Can you work these out from the model? Positions are in its coordinate system, mm. A direction names the side the tool comes from. Give positions to 0.01 mm unless a question says otherwise; leave off trailing zeros. Write each loop counter-clockwise with the first axis right and the second up, starting at its lowest first coordinate (ties: lowest second). Pieces come first, ordered by that corner, then holes.
from build123d import *

# Parameters (mm, degrees)
SKETCH1_R           = 2.3
BOSS_EXTRUDE1_DEPTH = 10


with BuildPart() as part:
    # Sketch1 → Boss-Extrude1 (new body)
    with BuildSketch(Plane.XY):
        with BuildLine():
            Line((14.271948898, -9.838051102), (14.061948898, -9.628051102))
            Line((14.061948898, -9.628051102), (14.271948898, -9.418051102))
            Line((14.271948898, -9.418051102), (14.271948898, -6.788711274))
            Line((14.271948898, -6.788711274), (16.932609069, -4.128051102))
            Line((16.932609069, -4.128051102), (18.571948898, -4.128051102))
            Line((18.571948898, -4.128051102), (18.571948898, -6.233051102))
            Line((18.571948898, -6.233051102), (19.186948898, -6.233051102))
            Line((19.186948898, -6.233051102), (20.371948898, -5.048051102))
            Line((20.371948898, -5.048051102), (20.371948898, 5.791948898))
            Line((20.371948898, 5.791948898), (19.186948898, 6.976948898))
            Line((19.186948898, 6.976948898), (18.571948898, 6.976948898))
            Line((18.571948898, 6.976948898), (18.571948898, 4.871948898))
            Line((18.571948898, 4.871948898), (16.932609069, 4.871948898))
            Line((16.932609069, 4.871948898), (14.271948898, 7.532609069))
            Line((14.271948898, 7.532609069), (14.271948898, 10.161948898))
            Line((14.271948898, 10.161948898), (14.061948898, 10.371948898))
            Line((14.061948898, 10.371948898), (14.271948898, 10.581948898))
            Line((14.271948898, 10.581948898), (14.271948898, 13.211288726))
            Line((14.271948898, 13.211288726), (16.932609069, 15.871948898))
            Line((16.932609069, 15.871948898), (18.571948898, 15.871948898))
            Line((18.571948898, 15.871948898), (18.571948898, 13.766948898))
            Line((18.571948898, 13.766948898), (19.186948898, 13.766948898))
            Line((19.186948898, 13.766948898), (20.371948898, 14.951948898))
            Line((20.371948898, 14.951948898), (20.371948898, 18.871948898))
            ThreePointArc((20.371948898, 18.871948898), (19.932609069, 19.932609069), (18.871948898, 20.371948898))
            Line((18.871948898, 20.371948898), (14.951948898, 20.371948898))
            Line((14.951948898, 20.371948898), (13.766948898, 19.186948898))
            Line((13.766948898, 19.186948898), (13.766948898, 18.571948898))
            Line((13.766948898, 18.571948898), (15.871948898, 18.571948898))
            Line((15.871948898, 18.571948898), (15.871948898, 16.932609069))
            Line((15.871948898, 16.932609069), (13.211288726, 14.271948898))
            Line((13.211288726, 14.271948898), (10.581948898, 14.271948898))
            Line((10.581948898, 14.271948898), (10.371948898, 14.061948898))
            Line((10.371948898, 14.061948898), (10.161948898, 14.271948898))
            Line((10.161948898, 14.271948898), (7.532609069, 14.271948898))
            Line((7.532609069, 14.271948898), (4.871948898, 16.932609069))
            Line((4.871948898, 16.932609069), (4.871948898, 18.571948898))
            Line((4.871948898, 18.571948898), (6.976948898, 18.571948898))
            Line((6.976948898, 18.571948898), (6.976948898, 19.186948898))
            Line((6.976948898, 19.186948898), (5.791948898, 20.371948898))
            Line((5.791948898, 20.371948898), (-5.048051102, 20.371948898))
            Line((-5.048051102, 20.371948898), (-6.233051102, 19.186948898))
            Line((-6.233051102, 19.186948898), (-6.233051102, 18.571948898))
            Line((-6.233051102, 18.571948898), (-4.128051102, 18.571948898))
            Line((-4.128051102, 18.571948898), (-4.128051102, 16.932609069))
            Line((-4.128051102, 16.932609069), (-6.788711274, 14.271948898))
            Line((-6.788711274, 14.271948898), (-9.418051102, 14.271948898))
            Line((-9.418051102, 14.271948898), (-9.628051102, 14.061948898))
            Line((-9.628051102, 14.061948898), (-9.838051102, 14.271948898))
            Line((-9.838051102, 14.271948898), (-12.467390931, 14.271948898))
            Line((-12.467390931, 14.271948898), (-15.128051102, 16.932609069))
            Line((-15.128051102, 16.932609069), (-15.128051102, 18.571948898))
            Line((-15.128051102, 18.571948898), (-13.023051102, 18.571948898))
            Line((-13.023051102, 18.571948898), (-13.023051102, 19.186948898))
            Line((-13.023051102, 19.186948898), (-14.208051102, 20.371948898))
            Line((-14.208051102, 20.371948898), (-18.128051102, 20.371948898))
            ThreePointArc((-18.128051102, 20.371948898), (-19.188711274, 19.932609069), (-19.628051102, 18.871948898))
            Line((-19.628051102, 18.871948898), (-19.628051102, 14.951948898))
            Line((-19.628051102, 14.951948898), (-18.443051102, 13.766948898))
            Line((-18.443051102, 13.766948898), (-17.828051102, 13.766948898))
            Line((-17.828051102, 13.766948898), (-17.828051102, 15.871948898))
            Line((-17.828051102, 15.871948898), (-16.188711274, 15.871948898))
            Line((-16.188711274, 15.871948898), (-13.528051102, 13.211288726))
            Line((-13.528051102, 13.211288726), (-13.528051102, 10.581948898))
            Line((-13.528051102, 10.581948898), (-13.318051102, 10.371948898))
            Line((-13.318051102, 10.371948898), (-13.528051102, 10.161948898))
            Line((-13.528051102, 10.161948898), (-13.528051102, 7.532609069))
            Line((-13.528051102, 7.532609069), (-16.188711274, 4.871948898))
            Line((-16.188711274, 4.871948898), (-17.828051102, 4.871948898))
            Line((-17.828051102, 4.871948898), (-17.828051102, 6.976948898))
            Line((-17.828051102, 6.976948898), (-18.443051102, 6.976948898))
            Line((-18.443051102, 6.976948898), (-19.628051102, 5.791948898))
            Line((-19.628051102, 5.791948898), (-19.628051102, -5.048051102))
            Line((-19.628051102, -5.048051102), (-18.443051102, -6.233051102))
            Line((-18.443051102, -6.233051102), (-17.828051102, -6.233051102))
            Line((-17.828051102, -6.233051102), (-17.828051102, -4.128051102))
            Line((-17.828051102, -4.128051102), (-16.188711274, -4.128051102))
            Line((-16.188711274, -4.128051102), (-13.528051102, -6.788711274))
            Line((-13.528051102, -6.788711274), (-13.528051102, -9.418051102))
            Line((-13.528051102, -9.418051102), (-13.318051102, -9.628051102))
            Line((-13.318051102, -9.628051102), (-13.528051102, -9.838051102))
            Line((-13.528051102, -9.838051102), (-13.528051102, -12.467390931))
            Line((-13.528051102, -12.467390931), (-16.188711274, -15.128051102))
            Line((-16.188711274, -15.128051102), (-17.828051102, -15.128051102))
            Line((-17.828051102, -15.128051102), (-17.828051102, -13.023051102))
            Line((-17.828051102, -13.023051102), (-18.443051102, -13.023051102))
            Line((-18.443051102, -13.023051102), (-19.628051102, -14.208051102))
            Line((-19.628051102, -14.208051102), (-19.628051102, -18.128051102))
            ThreePointArc((-19.628051102, -18.128051102), (-19.188711274, -19.188711274), (-18.128051102, -19.628051102))
            Line((-18.128051102, -19.628051102), (-14.208051102, -19.628051102))
            Line((-14.208051102, -19.628051102), (-13.023051102, -18.443051102))
            Line((-13.023051102, -18.443051102), (-13.023051102, -17.828051102))
            Line((-13.023051102, -17.828051102), (-15.128051102, -17.828051102))
            Line((-15.128051102, -17.828051102), (-15.128051102, -16.188711274))
            Line((-15.128051102, -16.188711274), (-12.467390931, -13.528051102))
            Line((-12.467390931, -13.528051102), (-9.838051102, -13.528051102))
            Line((-9.838051102, -13.528051102), (-9.628051102, -13.318051102))
            Line((-9.628051102, -13.318051102), (-9.418051102, -13.528051102))
            Line((-9.418051102, -13.528051102), (-6.788711274, -13.528051102))
            Line((-6.788711274, -13.528051102), (-4.128051102, -16.188711274))
            Line((-4.128051102, -16.188711274), (-4.128051102, -17.828051102))
            Line((-4.128051102, -17.828051102), (-6.233051102, -17.828051102))
            Line((-6.233051102, -17.828051102), (-6.233051102, -18.443051102))
            Line((-6.233051102, -18.443051102), (-5.048051102, -19.628051102))
            Line((-5.048051102, -19.628051102), (5.791948898, -19.628051102))
            Line((5.791948898, -19.628051102), (6.976948898, -18.443051102))
            Line((6.976948898, -18.443051102), (6.976948898, -17.828051102))
            Line((6.976948898, -17.828051102), (4.871948898, -17.828051102))
            Line((4.871948898, -17.828051102), (4.871948898, -16.188711274))
            Line((4.871948898, -16.188711274), (7.532609069, -13.528051102))
            Line((7.532609069, -13.528051102), (10.161948898, -13.528051102))
            Line((10.161948898, -13.528051102), (10.371948898, -13.318051102))
            Line((10.371948898, -13.318051102), (10.581948898, -13.528051102))
            Line((10.581948898, -13.528051102), (13.211288726, -13.528051102))
            Line((13.211288726, -13.528051102), (15.871948898, -16.188711274))
            Line((15.871948898, -16.188711274), (15.871948898, -17.828051102))
            Line((15.871948898, -17.828051102), (13.766948898, -17.828051102))
            Line((13.766948898, -17.828051102), (13.766948898, -18.443051102))
            Line((13.766948898, -18.443051102), (14.951948898, -19.628051102))
            Line((14.951948898, -19.628051102), (18.871948898, -19.628051102))
            ThreePointArc((18.871948898, -19.628051102), (19.932609069, -19.188711274), (20.371948898, -18.128051102))
            Line((20.371948898, -18.128051102), (20.371948898, -14.208051102))
            Line((20.371948898, -14.208051102), (19.186948898, -13.023051102))
            Line((19.186948898, -13.023051102), (18.571948898, -13.023051102))
            Line((18.571948898, -13.023051102), (18.571948898, -15.128051102))
            Line((18.571948898, -15.128051102), (16.932609069, -15.128051102))
            Line((16.932609069, -15.128051102), (14.271948898, -12.467390931))
            Line((14.271948898, -12.467390931), (14.271948898, -9.838051102))
        make_face()
        with Locations((-9.628051102, -9.628051102)):
            Circle(SKETCH1_R, mode=Mode.SUBTRACT)
        with Locations((10.371948898, -9.628051102)):
            Circle(SKETCH1_R, mode=Mode.SUBTRACT)
        with Locations((10.371948898, 10.371948898)):
            Circle(SKETCH1_R, mode=Mode.SUBTRACT)
        with Locations((-9.628051102, 10.371948898)):
            Circle(SKETCH1_R, mode=Mode.SUBTRACT)
        Polygon((-12.467390931, 6.471948898), (-6.788711274, 6.471948898), (-5.728051102, 7.532609069), (-5.728051102, 13.211288726), (-2.328051102, 16.611288726), (-2.328051102, 18.571948898), (3.071948898, 18.571948898), (3.071948898, 16.611288726), (6.471948898, 13.211288726), (6.471948898, 7.532609069), (7.532609069, 6.471948898), (13.211288726, 6.471948898), (16.611288726, 3.071948898), (18.571948898, 3.071948898), (18.571948898, -2.328051102), (16.611288726, -2.328051102), (13.211288726, -5.728051102), (7.532609069, -5.728051102), (6.471948898, -6.788711274), (6.471948898, -12.467390931), (3.071948898, -15.867390931), (3.071948898, -17.828051102), (-2.328051102, -17.828051102), (-2.328051102, -15.867390931), (-5.728051102, -12.467390931), (-5.728051102, -6.788711274), (-6.788711274, -5.728051102), (-12.467390931, -5.728051102), (-15.867390931, -2.328051102), (-17.828051102, -2.328051102), (-17.828051102, 3.071948898), (-15.867390931, 3.071948898), align=None, mode=Mode.SUBTRACT)
    extrude(amount=BOSS_EXTRUDE1_DEPTH)


solid = part.part
(1) If we mould it in two halves opening along X, with no side actions, what happens to faces 3 (the face through (7.01, -6.25, 4.93)), 4 (the face through (20.372, 0, 5)), 5 (the face through (-19.044, 14.368, 4.93))? For each: +X half, -X half, draft (parallel to the pull), parting line (faces both ways), or undercut.
Returned:
face 3: undercut
face 4: +X half
face 5: -X half
(2) If I drill on L1, parallel to Y at x = -17, z = 6.5; L2, parallel to Y at x = 0.5, z = 4.25; L3, parallel to Y at x = 13, z = 7, over which ranges is the centre line in solid material (lowest first)?
Returned:
L1: y = -19.63 to -15.13, -4.13 to -2.33, 3.07 to 4.87, 15.87 to 20.37
L2: y = -19.63 to -17.83, 18.57 to 20.37
L3: y = -13.53 to -5.73, 6.47 to 14.27
(3) For faces 1 (the face through (15, -17.828, 5)), 2 (the face through (14.37, 19.79, 4.93)), which set-ups out of +Z, -Z, +X, -X, +Y, -Y let a thin tool reach every point of the face, with its end or its side?
Returned:
face 1: +Z, -Z
face 2: +Z, -Z, +Y
(4) Imagine slicing it at A-A, the plane y = 2.5. Write out the boundary of the cut face in (x, z), plus the area to 3 significant figures.
Returned:
outline: (-19.63, 0) - (-17.83, 0) - (-17.83, 10) - (-19.63, 10) - close; (18.57, 0) - (20.37, 0) - (20.37, 10) - (18.57, 10) - close
area: 36.0 mm2
(5) Imagine slicing it at C-C, the plane x = -11. Write out the boundary of the cut face in (y, z), plus the area to 3 significant figures.
Returned:
outline: (-13.53, 0) - (-11.47, 0) - (-11.47, 10) - (-13.53, 10) - close; (-7.78, 0) - (-5.73, 0) - (-5.73, 10) - (-7.78, 10) - close; (6.47, 0) - (8.53, 0) - (8.53, 10) - (6.47, 10) - close; (12.22, 0) - (14.27, 0) - (14.27, 10) - (12.22, 10) - close
area: 82.2 mm2
(6) Imagine slicing it at D-D, the plane z = 3.75. Give the number of separate pieces and of enclosed holes in the cut face, plus the area to 3 significant figures.
Returned:
separate pieces: 1
enclosed holes: 5
area: 458 mm2
(7) Will these pins go through, and if not, where does the flat tip stop? P1, Ø4.5, axis at y = -11, z = 6.5, coming from the -X side; P2, Ø1.5, axis at x = 16.5, y = -7, coming from the +Z side; P3, Ø1.3, axis at y = -8, z = 4, coming from the +X side; P4, Ø1.5, axis at x = 13.5, z = 2, coming from the +Y side.
Returned:
P1: stops at x = -18.67
P2: passes through
P3: stops at x = 14.27
P4: stops at y = 19.67
